Build history of the part. All positions in model axes, mm. A direction names the side the tool comes from. Round coordinates to 2 decimals unless told otherwise and drop trailing zeros. Loops run counter-clockwise (first coordinate to the right, second up) from the corner with the lowest first, then second, coordinate; pieces in that order, holes last. Notation, with made-up numbers: (-24, 13.25) - (-17, 13.25) arc R16 cw to (-17, 28.25) - close; hole circle Ø2 at (74, 74.5). An arc over 180 degrees is marked (long way). Put each result on its own line as item: value. Start each with the question number.
from build123d import *

# Parameters (mm, degrees)
SKETCH1_W           = 40
SKETCH1_H           = 29
BASE_FLANGE1_DEPTH  = 2
BREAK_CORNER1_START = -2
BREAK_CORNER1_DEPTH = 2
HEM2_START          = -19
HEM2_DEPTH          = 38
SKETCH10_W          = 1
SKETCH10_H          = 4.2
CUT_EXTRUDE1_DEPTH  = 10
SKETCH11_R          = 2
CUT_EXTRUDE2_DEPTH  = 2
CHAMFER1_SIZE       = 1


# Read off the part's stored shape, not the designer's step: Break-Corner1, Hem2
# Sheet-metal steps are written as plain solids
with BuildPart() as part:
    # Sketch1 → Base-Flange1 (new body)
    with BuildSketch(Plane(origin=(0, 0, 0), x_dir=(1, 0, 0), z_dir=(0, 1, 0))):
        Rectangle(SKETCH1_W, SKETCH1_H)
    extrude(amount=-BASE_FLANGE1_DEPTH)

    # Break-Corner1 outline → Break-Corner1 (cut)
    with BuildSketch(Plane(origin=(0, 0, 0), x_dir=(1, 0, 0), z_dir=(0, 1, 0)).offset(BREAK_CORNER1_START)):
        Polygon((-20, 14.5), (-20, 11.5), (-17, 14.5), align=None)
        Polygon((20, 14.5), (17, 14.5), (20, 11.5), align=None)
    extrude(amount=BREAK_CORNER1_DEPTH, mode=Mode.SUBTRACT)

    # Hem2 outline → Hem2 (add)
    with BuildSketch(Plane.YZ.offset(HEM2_START)):
        with BuildLine():
            Line((2.038247626, 11.843703978), (1.520609536, 9.911852325))
            ThreePointArc((1.520609536, 9.911852325), (6.518428366, 17.391616788), (-2, 14.5))
            Line((-2, 14.5), (0, 14.5))
            ThreePointArc((0, 14.5), (4.931721686, 16.17409393), (2.038247626, 11.843703978))
        make_face()
    extrude(amount=HEM2_DEPTH)

    # Sketch10 → Cut-Extrude1 (cut)
    with BuildSketch(Plane(origin=(0, 0, 0), x_dir=(1, 0, 0), z_dir=(0, 1, 0))):
        with Locations((19.5, -12.4)):
            Rectangle(SKETCH10_W, SKETCH10_H)
        with Locations((-19.5, -12.4)):
            Rectangle(SKETCH10_W, SKETCH10_H)
    extrude(amount=-CUT_EXTRUDE1_DEPTH, mode=Mode.SUBTRACT)

    # Sketch11 → Cut-Extrude2 (cut)
    with BuildSketch(Plane(origin=(0, 0, 0), x_dir=(1, 0, 0), z_dir=(0, 1, 0))):
        with Locations(Location((-15, 9.5, 0), (0, 0, 270))):
            Circle(SKETCH11_R)
        with Locations(Location((0, 7.5, 0), (0, 0, 270))):
            Circle(SKETCH11_R)
        with Locations(Location((15, 9.5, 0), (0, 0, 270))):
            Circle(SKETCH11_R)
    extrude(amount=-CUT_EXTRUDE2_DEPTH, mode=Mode.SUBTRACT)

    # Chamfer1
    chamfer1_edges = [part.edges().sort_by_distance(p)[0] for p in [
        (-15, 0, -11.5),
        (0, 0, -9.5),
        (15, 0, -11.5),
    ]]
    chamfer(chamfer1_edges, length=CHAMFER1_SIZE)


solid = part.part
1) Drill centre lines: line 1 (Z direction, x = 11.5, y = 2.75); line 2 (Y direction, x = 16, z = -4); line 3 (Z direction, x = 6, y = 3.5). Where is each one in solid material? Low to high. Write a range as [from, to].
2) Slice it at B-B, the plane y = 2.75. Write the cut outline in (x, z).
3) Slice it at A-A, the plane x = 15. Write the cut outline in (y, z).
4) Drop flat-ended pins along their axis: pin 1 Ø2 at (x, z) = (-2, 2.5) entering from +Y; pin 2 Ø4 at (x, z) = (-6, 12) entering from +Y. Give the stop position or say it passes through.
5) Slice it at C-C, the plane x = -6.5. Write the cut outline in (y, z), and give its area (3 significant figures).
6) Pull direction X, two halves, no side cores. Call faces 1 (the face through (-0.266, 6.617, 17.259)), 2 (the face through (-19, -0.4, 14.6)), 3 (the face through (16.983, -1.493, -9.76)): pulls with the +X half, pulls with the -X half, needs draft (parallel to the pull), parting line crosses it, or undercut.
7) Which spindle directions (+Z, -Z, +X, -X, +Y, -Y) get a long thin tool onto all of the face, cutting with end or side? Do faces 4 (the face through (-19.5, -1, 10.3)), 5 (the face through (-20, -1, 0)), 6 (the face through (-0.266, 1.783, 10.891)). Say none if no direction does.
8) Slice it at D-D, the plane y = 4.75. Write the cut outline in (x, z), and give its area (3 significant figures).
Taken from the geometry:
1. line 1: z = [9.75, 11.75], [17.25, 19.25]
1. line 2: y = [-2, 0]
1. line 3: z = [9.81, 11.85], [17.15, 19.19]
2. outline: (-19, 9.75) - (19, 9.75) - (19, 11.75) - (-19, 11.75) - close; (-19, 17.25) - (19, 17.25) - (19, 19.25) - (-19, 19.25) - close
3. outline: (-2, -14.5) - (0, -14.5) - (0, -12.5) - (-1, -11.5) - (-2, -11.5) - close; (-2, -7.5) - (-1, -7.5) - (0, -6.5) - (0, 14.5) arc R2.75 cw (long way) to (2.04, 11.84) - (1.52, 9.91) arc R4.75 ccw (long way) to (-2, 14.5) - close
4. pin 1: stops at y = 0
4. pin 2: stops at y = 7.47
5. outline: (-2, -14.5) - (0, -14.5) - (0, 14.5) arc R2.75 cw (long way) to (2.04, 11.84) - (1.52, 9.91) arc R4.75 ccw (long way) to (-2, 14.5) - close
5. area: 95.3 mm2
6. face 1: needs draft
6. face 2: pulls with the -X half
6. face 3: undercut
7. face 4: +Z, -X, +Y, -Y
7. face 5: +Z, -Z, -X, +Y, -Y
7. face 6: +X, -X
8. outline: (-19, 10.19) - (19, 10.19) - (19, 12.61) - (-19, 12.61) - close; (-19, 16.39) - (19, 16.39) - (19, 18.81) - (-19, 18.81) - close
8. area: 184 mm2
